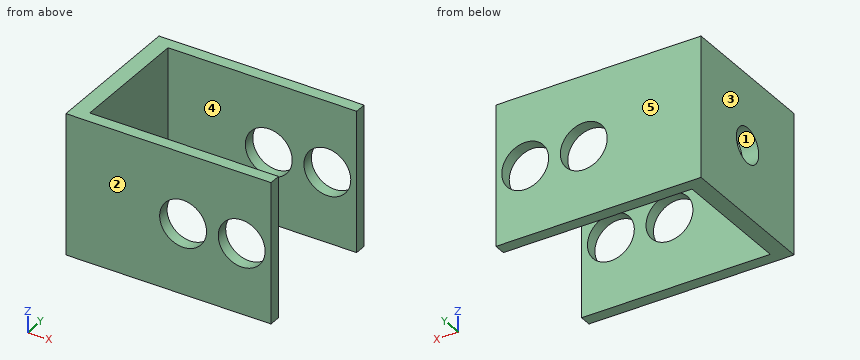
from build123d import *

# Parameters (mm, degrees)
BOSS_EXTRU_1_DEPTH      = 24
ENL_V_MAT_EXTRU_1_REACH = 40.823
ESQUISSE2_R             = 4
ENL_V_MAT_EXTRU_2_REACH = 46.241
ESQUISSE3_R             = 3


with BuildPart() as part:
    # Esquisse1 → Boss.-Extru.1 (new body)
    with BuildSketch(Plane.XY):
        Polygon((17.5, -10.5), (17.5, -12.5), (-17.5, -12.5), (-17.5, 12.5), (17.5, 12.5), (17.5, 10.5), (-14.7, 10.5), (-14.7, -10.5), align=None)
    extrude(amount=BOSS_EXTRU_1_DEPTH)

    # Enlèv. mat.-Extru.1: up to this face of the body (flat: up to its plane)
    enl_v_mat_extru_1_end = Plane(part.part.faces().sort_by_distance((0, -12.5, 12))[0])
    # Esquisse2 → Enlèv. mat.-Extru.1 (cut, up to the picked face)
    with BuildSketch(Plane(origin=(0, 12.5, 0), x_dir=(1, 0, 0), z_dir=(0, 1, 0)), mode=Mode.PRIVATE) as enl_v_mat_extru_1_sk1:
        with Locations(Location((12.5, -12, 0), (0, 0, 270))):
            Circle(ESQUISSE2_R)
    enl_v_mat_extru_1_tool1 = split(extrude(enl_v_mat_extru_1_sk1.sketch, amount=-ENL_V_MAT_EXTRU_1_REACH, mode=Mode.PRIVATE), bisect_by=enl_v_mat_extru_1_end, keep=Keep.BOTH, mode=Mode.PRIVATE)
    # Esquisse2 → Enlèv. mat.-Extru.1 (cut, up to the picked face)
    with BuildSketch(Plane(origin=(0, 12.5, 0), x_dir=(1, 0, 0), z_dir=(0, 1, 0)), mode=Mode.PRIVATE) as enl_v_mat_extru_1_sk2:
        with Locations(Location((2.5, -12, 0), (0, 0, 270))):
            Circle(ESQUISSE2_R)
    enl_v_mat_extru_1_tool2 = split(extrude(enl_v_mat_extru_1_sk2.sketch, amount=-ENL_V_MAT_EXTRU_1_REACH, mode=Mode.PRIVATE), bisect_by=enl_v_mat_extru_1_end, keep=Keep.BOTH, mode=Mode.PRIVATE)
    add(enl_v_mat_extru_1_tool1.solids().sort_by(Axis((12.5, 12.5, 12), (0, -1, 0)))[0], mode=Mode.SUBTRACT)
    add(enl_v_mat_extru_1_tool2.solids().sort_by(Axis((2.5, 12.5, 12), (0, -1, 0)))[0], mode=Mode.SUBTRACT)

    # Esquisse3 → Enlèv. mat.-Extru.2 (cut, up to next)
    with BuildSketch(Plane.ZY.offset(17.5), mode=Mode.PRIVATE) as enl_v_mat_extru_2_sk1:
        with Locations(Location((12, 0, 0), (0, 0, 270))):
            Circle(ESQUISSE3_R)
    enl_v_mat_extru_2_tool1 = extrude(enl_v_mat_extru_2_sk1.sketch, amount=-ENL_V_MAT_EXTRU_2_REACH, mode=Mode.PRIVATE) & part.part
    add(enl_v_mat_extru_2_tool1.solids().sort_by_distance((-17.5, 0, 12))[0], mode=Mode.SUBTRACT)


solid = part.part
Can you work these out from the model? Positions are in its coordinate system, mm. Face numbers are marked on the shaded views. A direction names the side the tool comes from. Give positions to 0.01 mm unless a question says otherwise; leave off trailing zeros. Order: outer loops, then holes, each group sorted by start corner. A loop starts at its lowest first (then second) coordinate and runs counter-clockwise, first axis right, second up. Notation, with made-up numbers: M -12,43.25 L 21,43.25 A17 ccw 21,56.25 Z; hole C 81.25,35 d1. An arc over 180 degrees is marked long. Use a Markdown table: item, result. Add a question column.
Item 1: We'd pull the mould along Y, two halves only. Please class the marked faces 1, 2 and 3: +Y half, -Y half, draft (parallel to the pull), parting line (faces both ways), or undercut.
Item 2: Suppose I cut it at B-B (z = 12). List the corners of the cut face in (x, y) for me.
Item 3: Suppose I cut it at D-D (x = 12.5). List the corners of the cut face in (y, z) for me.
Item 4: Will this pin go through, and if not, where does the flat tip stop? pin 1 (8 mm diameter, centred on y = 0, z = 12, fed in from +X).
Item 5: Suppose I cut it at C-C (x = -7). List the corners of the cut face in (y, z) for me, then the cut area to 3 significant figures.
Item 6: Suppose I cut it at A-A (y = 0). List the corners of the cut face in (x, z) for me, then the cut area to 3 significant figures.
Item 7: For the marked faces 4 and 5, which set-ups out of +Z, -Z, +X, -X, +Y, -Y let a thin tool reach every point of the face, with its end or its side?
Item 8: If I drill on L1, parallel to X at y = -11.9, z = 12; L2, parallel to Y at x = 0.5, z = 6.5; L3, parallel to X at y = -9, z = 2.5, over which ranges is the centre line in solid material (lowest first)? Write a range as [from, to].
Answer sheet:
| question | item | result |
|---|---|---|
| 1 | face 1 | undercut |
| 1 | face 2 | -Y half |
| 1 | face 3 | draft |
| 2 | outline | M -17.5,-12.5 L -1.5,-12.5 L -1.5,-10.5 L -14.7,-10.5 L -14.7,-3 L -17.5,-3 Z; M -17.5,3 L -14.7,3 L -14.7,10.5 L -1.5,10.5 L -1.5,12.5 L -17.5,12.5 Z; M 6.5,-12.5 L 8.5,-12.5 L 8.5,-10.5 L 6.5,-10.5 Z; M 6.5,10.5 L 8.5,10.5 L 8.5,12.5 L 6.5,12.5 Z; M 16.5,-12.5 L 17.5,-12.5 L 17.5,-10.5 L 16.5,-10.5 Z; M 16.5,10.5 L 17.5,10.5 L 17.5,12.5 L 16.5,12.5 Z |
| 3 | outline | M -12.5,0 L -10.5,0 L -10.5,8 L -12.5,8 Z; M -12.5,16 L -10.5,16 L -10.5,24 L -12.5,24 Z; M 10.5,0 L 12.5,0 L 12.5,8 L 10.5,8 Z; M 10.5,16 L 12.5,16 L 12.5,24 L 10.5,24 Z |
| 4 | pin 1 | stops at x = -14.7 |
| 5 | outline | M -12.5,0 L -10.5,0 L -10.5,24 L -12.5,24 Z; M 10.5,0 L 12.5,0 L 12.5,24 L 10.5,24 Z |
| 5 | area | 96.0 mm² |
| 6 | outline | M -17.5,0 L -14.7,0 L -14.7,9 L -17.5,9 Z; M -17.5,15 L -14.7,15 L -14.7,24 L -17.5,24 Z |
| 6 | area | 50.4 mm² |
| 7 | face 4 | +Z, -Z, +X |
| 7 | face 5 | +Z, -Z, +X, -X, +Y |
| 8 | L1 | x = [-17.5, -1.5], [6.5, 8.5], [16.5, 17.5] |
| 8 | L2 | y = [-12.5, -10.5], [10.5, 12.5] |
| 8 | L3 | x = [-17.5, -14.7] |
